```python
from build123d import *

# Parameters (mm, degrees)
F0_W     = 101.6
F0_H     = 50.8
F1_DEPTH = 12.7
F2_D     = 2
F2_DEPTH = 14.1986
F2_TIP   = 0.600860619
F3_D     = 2
F3_DEPTH = 14.1986
F3_TIP   = 0.600860619
F4_D     = 2
F4_DEPTH = 14.1986
F4_TIP   = 0.600860619
F5_D     = 2
F5_DEPTH = 14.2
F5_TIP   = 0.600860619


with BuildPart() as f1:
    # F0 (on Top) → F1 (new body)
    with BuildSketch(Plane.XY):
        with Locations((0, -0.6499526367)):
            Rectangle(F0_W, F0_H)
        with BuildLine():
            ThreePointArc((-48.26, 17.0429494041), (-43.933302429, 17.85827907), (-43.2645819675, 22.2100473633))
            Line((-43.2645819675, 22.2100473633), (43.0625333975, 22.2100473633))
            ThreePointArc((43.0625333975, 22.2100473633), (43.810791793, 17.7784065979), (48.26, 17.1428935527))
            Line((48.26, 17.1428935527), (48.26, -18.3574629872))
            ThreePointArc((48.26, -18.3574629872), (43.7766277668, -19.0267059263), (43.1065444682, -23.5099526367))
            Line((43.1065444682, -23.5099526367), (-43.1065444682, -23.5099526367))
            ThreePointArc((-43.1065444682, -23.5099526367), (-43.7766277668, -19.0267059263), (-48.26, -18.3574629872))
            Line((-48.26, -18.3574629872), (-48.26, 17.0429494041))
        make_face(mode=Mode.SUBTRACT)
    extrude(amount=F1_DEPTH)

    # F2
    with Locations(Plane(origin=(0, 0, 0), x_dir=(1, 0, 0), z_dir=(0, 0, -1))):
        with Locations((46.4704521, -20.5064658076)):
            Hole(F2_D / 2, depth=F2_DEPTH)
            with Locations((0, 0, -(F2_DEPTH + F2_TIP / 2))):  # 118° drill point
                Cone(0, F2_D / 2, F2_TIP, mode=Mode.SUBTRACT)

    # F3
    with Locations(Plane(origin=(0, 0, 0), x_dir=(1, 0, 0), z_dir=(0, 0, -1))):
        with Locations((-46.4704521, 21.7210352421)):
            Hole(F3_D / 2, depth=F3_DEPTH)
            with Locations((0, 0, -(F3_DEPTH + F3_TIP / 2))):  # 118° drill point
                Cone(0, F3_D / 2, F3_TIP, mode=Mode.SUBTRACT)

    # F4
    with Locations(Plane(origin=(0, 0, 0), x_dir=(1, 0, 0), z_dir=(0, 0, -1))):
        with Locations((46.4704521, 21.7210352421)):
            Hole(F4_D / 2, depth=F4_DEPTH)
            with Locations((0, 0, -(F4_DEPTH + F4_TIP / 2))):  # 118° drill point
                Cone(0, F4_D / 2, F4_TIP, mode=Mode.SUBTRACT)

    # F5
    with Locations(Plane(origin=(0, 0, 0), x_dir=(1, 0, 0), z_dir=(0, 0, -1))):
        with Locations((-46.67250067, -20.5064658076)):
            Hole(F5_D / 2, depth=F5_DEPTH)
            with Locations((0, 0, -(F5_DEPTH + F5_TIP / 2))):  # 118° drill point
                Cone(0, F5_D / 2, F5_TIP, mode=Mode.SUBTRACT)


solid = f1.part
```
Input: part model. Units: mm. Frame: model coordinates. A direction names the side the tool comes from. Round coordinates to 2 decimals unless told otherwise and drop trailing zeros. Write each loop counter-clockwise with the first axis right and the second up, starting at its lowest first coordinate (ties: lowest second). Pieces come first, ordered by that corner, then holes. Notation, with made-up numbers: (-9, 57) - (33, 57) arc R20 ccw to (33, 73) - close; hole circle Ø1 at (-11, -13). An arc over 180 degrees is marked (long way). Write item = value, one per line.
(1) Contact query for a flat-ended pin moving along its axis: pin 1 Ø1.2 at (x, y) = (46.47, 20.51) entering from -Z. Output: stop coordinate, or through.
Geometry check:
pin_1 = through
(2) Section query C-C on z = 3.5. Output: boundary loops of the cut face in (x, y).
Geometry check:
outline = (-50.8, -26.05) - (50.8, -26.05) - (50.8, 24.75) - (-50.8, 24.75) - close; hole (-48.26, -18.36) arc R3.81 cw to (-43.11, -23.51) - (43.11, -23.51) arc R3.81 cw to (48.26, -18.36) - (48.26, 17.14) arc R3.81 cw to (43.06, 22.21) - (-43.26, 22.21) arc R3.81 cw to (-48.26, 17.04) - close; hole circle Ø2 at (-46.67, 20.51); hole circle Ø2 at (-46.47, -21.72); hole circle Ø2 at (46.47, -21.72); hole circle Ø2 at (46.47, 20.51)
(3) Pull-direction query (X, two-part tool) for faces 1 (the flat face through (50.8, -1, 6)), 2 (the flat face through (0, 24, 12.7)), 3 (the flat face through (-48.26, -1, 6)); classes: +X half, -X half, draft (parallel to the pull), parting line (faces both ways), or undercut.
Geometry check:
face_1 = +X half
face_2 = draft
face_3 = undercut
(4) Section query A-A on x = 14. Output: boundary loops of the cut face in (y, z).
Geometry check:
outline = (-26.05, 0) - (-23.51, 0) - (-23.51, 12.7) - (-26.05, 12.7) - close; (22.21, 0) - (24.75, 0) - (24.75, 12.7) - (22.21, 12.7) - close
(5) Section query B-B on y = 10. Output: boundary loops of the cut face in (x, z).
Geometry check:
outline = (-50.8, 0) - (-48.26, 0) - (-48.26, 12.7) - (-50.8, 12.7) - close; (48.26, 0) - (50.8, 0) - (50.8, 12.7) - (48.26, 12.7) - close
(6) Access query for faces 4 (the flat face through (-1, 24.75, 6)), 5 (the flat face through (-1, 22.21, 6)). Directions: +Z, -Z, +X, -X, +Y, -Y. A direction counts if a zero-diameter tool reaches every point of the face in a straight line with its end or side. Return the directions, or none.
Geometry check:
face_4 = +Z, -Z, +X, -X, +Y
face_5 = +Z, -Z
(7) Material intervals for probe 1 along X at (y, z) = (20.5, 3.5); probe 2 along Y at (x, z) = (-20.5, 6.5); probe 3 along X at (y, z) = (-4.5, 2), sorted ascending.
Geometry check:
probe_1 = -50.8 to -47.67, -45.67 to -42.86, 42.66 to 45.47, 47.47 to 50.8
probe_2 = -26.05 to -23.51, 22.21 to 24.75
probe_3 = -50.8 to -48.26, 48.26 to 50.8
